Check sheet for the modelled part. Datum: model origin and axes. Units: mm. Face numbers are marked on the shaded views. A direction names the side the tool comes from. Coordinates: 2 decimals unless noted, no trailing zeros. Order: outer loops, then holes, each group sorted by start corner. A loop starts at its lowest first (then second) coordinate and runs counter-clockwise, first axis right, second up.
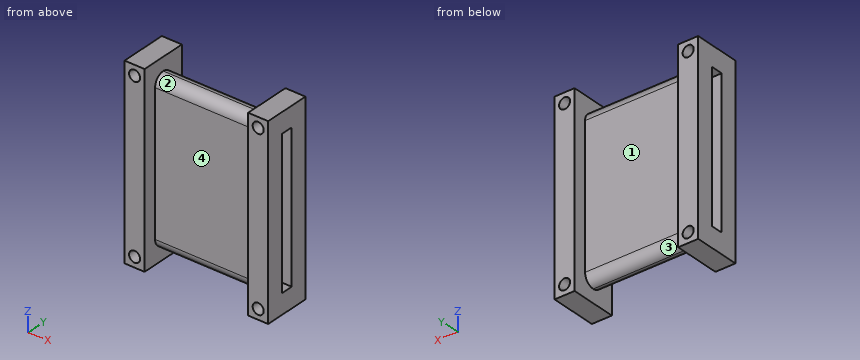
from build123d import *

# Parameters (mm, degrees)
SKETCH1_W           = 46.4
SKETCH1_H           = 5.9
SKETCH1_W_2         = 42.4
SKETCH1_H_2         = 3.5
BOSS_EXTRUDE1_DEPTH = 30
FILLET2_R           = 3
SKETCH2_W           = 54
SKETCH2_H           = 13.5
SKETCH2_W_2         = 42.4
SKETCH2_H_2         = 3.5
BOSS_EXTRUDE2_DEPTH = 5.8
SKETCH3_W           = 54
SKETCH3_H           = 13.5
SKETCH3_W_2         = 42.4
SKETCH3_H_2         = 3.5
BOSS_EXTRUDE3_DEPTH = 5.8
SKETCH4_R           = 1.6
CUT_EXTRUDE1_DEPTH  = 64.118380841


with BuildPart() as part:
    # Sketch1 → Boss-Extrude1 (new body)
    with BuildSketch(Plane(origin=(0, 0, 0), x_dir=(0, 0, -1), z_dir=(1, 0, 0))):
        with Locations((23.2, 2.95)):
            Rectangle(SKETCH1_W, SKETCH1_H)
        with Locations((23.2, 2.95)):
            Rectangle(SKETCH1_W_2, SKETCH1_H_2, mode=Mode.SUBTRACT)
    extrude(amount=BOSS_EXTRUDE1_DEPTH)

    # Fillet2
    # the kernel refuses this fillet: 3 mm, written as the material it takes off along each edge
    with BuildSketch(Plane(origin=(-7.5, 0, -46.4), x_dir=(0, 0, 1), z_dir=(1, 0, 0)), Plane(origin=(-7.5, 5.9, 0), x_dir=(0, 0, -1), z_dir=(1, 0, 0)), Plane(origin=(-7.5, 5.9, -46.4), x_dir=(0, -1, 0), z_dir=(1, 0, 0))) as fillet2_piece_1:
        with BuildLine():
            CenterArc((FILLET2_R, -FILLET2_R), FILLET2_R, 90, 90)
            Line((0, -FILLET2_R), (0, 0))
            Line((0, 0), (FILLET2_R, 0))
        make_face()
    extrude(amount=45, mode=Mode.SUBTRACT)
    with BuildSketch(Plane(origin=(-7.5, 0, 0), x_dir=(0, 0, -1), z_dir=(1, 0, 0))) as fillet2_piece_2:
        with BuildLine():
            CenterArc((FILLET2_R, FILLET2_R), FILLET2_R, 180, 90)
            Line((0, FILLET2_R), (0, 0))
            Line((0, 0), (FILLET2_R, 0))
        make_face()
    extrude(amount=45, mode=Mode.SUBTRACT)

    # Sketch2 → Boss-Extrude2 (add)
    with BuildSketch(Plane(origin=(30, 0, 0), x_dir=(0, 0, -1), z_dir=(1, 0, 0))):
        with Locations((23.2, 2.95)):
            Rectangle(SKETCH2_W, SKETCH2_H)
        with Locations((23.2, 2.95)):
            Rectangle(SKETCH2_W_2, SKETCH2_H_2, mode=Mode.SUBTRACT)
    extrude(amount=BOSS_EXTRUDE2_DEPTH)

    # Sketch3 → Boss-Extrude3 (add)
    with BuildSketch(Plane.ZY):
        with Locations((-23.2, 2.95)):
            Rectangle(SKETCH3_W, SKETCH3_H)
        with Locations((-23.2, 2.95)):
            Rectangle(SKETCH3_W_2, SKETCH3_H_2, mode=Mode.SUBTRACT)
    extrude(amount=BOSS_EXTRUDE3_DEPTH)

    # Sketch4 → Cut-Extrude1 (cut, through all)
    with BuildSketch(Plane(origin=(0, 9.7, 0), x_dir=(1, 0, 0), z_dir=(0, 1, 0))):
        with Locations(Location((-2.9, 47.3, 0), (0, 0, 270))):
            Circle(SKETCH4_R)
        with Locations(Location((32.9, 47.3, 0), (0, 0, 270))):
            Circle(SKETCH4_R)
        with Locations(Location((-2.9, -0.9, 0), (0, 0, 270))):
            Circle(SKETCH4_R)
        with Locations(Location((32.9, -0.9, 0), (0, 0, 270))):
            Circle(SKETCH4_R)
    extrude(amount=-CUT_EXTRUDE1_DEPTH, mode=Mode.SUBTRACT)


solid = part.part
(1) Cross-section at C-C (z = -28). Enter the section's corners in (x, y).
Filled in:
outline: (-5.8, -3.8) - (0, -3.8) - (0, 0) - (30, 0) - (30, -3.8) - (35.8, -3.8) - (35.8, 1.2) - (-5.8, 1.2) - close; (-5.8, 4.7) - (35.8, 4.7) - (35.8, 9.7) - (30, 9.7) - (30, 5.9) - (0, 5.9) - (0, 9.7) - (-5.8, 9.7) - close
(2) Tool access check on the marked faces 1, 2, 3 and 4. Record the directions out of +Z, -Z, +X, -X, +Y, -Y that give a thin tool (end or side, any length) a straight path to the whole face; none if there is none.
Filled in:
face 1: +Z, -Z, +Y
face 2: +Z, -Y
face 3: -Z, +Y
face 4: +Z, -Z, -Y
(3) Cross-section at B-B (x = 32.9). Enter the section's corners in (y, z), and give its area (3 significant figures).
Filled in:
outline: (-3.8, -50.2) - (9.7, -50.2) - (9.7, -48.9) - (-3.8, -48.9) - close; (-3.8, -45.7) - (9.7, -45.7) - (9.7, -0.7) - (-3.8, -0.7) - close; (-3.8, 2.5) - (9.7, 2.5) - (9.7, 3.8) - (-3.8, 3.8) - close; hole (1.2, -44.4) - (4.7, -44.4) - (4.7, -2) - (1.2, -2) - close
area: 494 mm2
(4) Cross-section at D-D (x = 25). Enter the section's corners in (y, z).
Filled in:
outline: (0, -43.4) arc R3 ccw to (2.95, -46.4) arc R3 ccw to (5.9, -43.4) - (5.9, -3) arc R3 ccw to (2.95, 0) arc R3 ccw to (0, -3) - close; hole (1.2, -44.4) - (4.7, -44.4) - (4.7, -2) - (1.2, -2) - close
(5) Cross-section at A-A (y = -1). Enter the section's corners in (x, z), and give its area (3 significant figures).
Filled in:
outline: (-5.8, -50.2) - (0, -50.2) - (0, 3.8) - (-5.8, 3.8) - close; (30, -50.2) - (35.8, -50.2) - (35.8, 3.8) - (30, 3.8) - close; hole circle Ø3.2 at (-2.9, -47.3); hole circle Ø3.2 at (-2.9, 0.9); hole circle Ø3.2 at (32.9, -47.3); hole circle Ø3.2 at (32.9, 0.9)
area: 594 mm2
(6) Go/stop test with flat-tipped pins: P1, Ø2, axis at x = 23.5, y = 7, coming from the -Z side; P2, Ø1.8, axis at x = 17.5, y = 2.5, coming from the -Z side; P3, Ø3, axis at x = 15, y = 2, coming from the +Z side; P4, Ø9, axis at x = 13, z = -25.5, coming from the -Y side. Record where each tip stops, or that it passes through.
Filled in:
P1: passes through
P2: stops at z = -46.4
P3: stops at z = 0
P4: stops at y = 0
(7) Thickness scan on probe 1 along X at (y, z) = (1.5, -47.3); probe 2 along Y at (x, z) = (-1.5, -19.5); probe 3 along X at (y, z) = (-1.5, 0). Record the ranges inside material, lowest first.
Filled in:
probe 1: x = -5.8 to -4.5, -1.3 to 0, 30 to 31.3, 34.5 to 35.8
probe 2: y = -3.8 to 1.2, 4.7 to 9.7
probe 3: x = -5.8 to -4.22, -1.58 to 0, 30 to 31.58, 34.22 to 35.8
